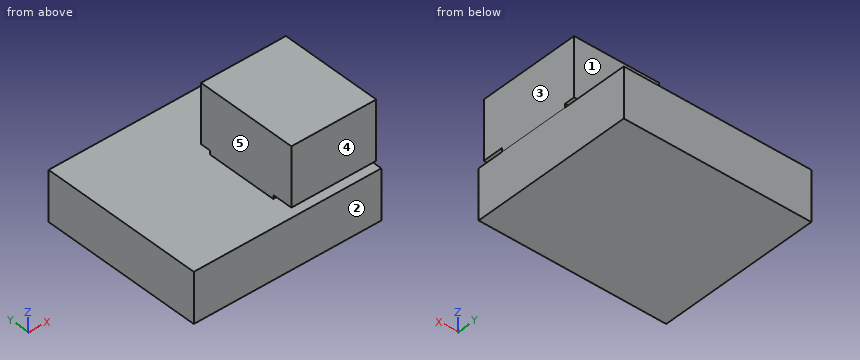
```python
from build123d import *

# Parameters (mm, degrees)
F0_W     = 95.4314470291
F0_H     = 83.3230912685
F1_DEPTH = 25.4
F2_W     = 36.3040966913
F2_H     = 16.6404070333
F3_DEPTH = 43.18


with BuildPart() as f1:
    # F0 (on Top) → F1 (new body)
    with BuildSketch(Plane.XY):
        with Locations((-4.4675134122, -1.5228800476)):
            Rectangle(F0_W, F0_H)
    extrude(amount=F1_DEPTH)

    # F2 (on Right) → F3 (join)
    with BuildSketch(Plane.YZ):
        Polygon((-40.3462946415, 57.2510994971), (-40.3462946415, 27.3906495422), (-29.9596916884, 27.3906495422), (6.3444050029, 27.3906495422), (11.5222530439, 27.3906495422), (11.5222530439, 57.2510994971), align=None)
        with Locations((-11.8076433428, 19.0704460256)):
            Rectangle(F2_W, F2_H)
    extrude(amount=F3_DEPTH)


solid = f1.part
```
Check sheet for the modelled part. Datum: model origin and axes. Units: mm. Face numbers are marked on the shaded views. A direction names the side the tool comes from. Round coordinates to 2 decimals unless told otherwise and drop trailing zeros. Order: outer loops, then holes, each group sorted by start corner. A loop starts at its lowest first (then second) coordinate and runs counter-clockwise, first axis right, second up. Notation, with made-up numbers: M -38.5,-27.5 L 11.5,-27.5 A29 ccw 11.5,1.5 Z; hole C -4.75,27.5 d5. An arc over 180 degrees is marked long. Answer in a Markdown table with one row per item.
(1) Set-up check for the marked faces 1 and 2: record each of +Z, -Z, +X, -X, +Y, -Y from which the full face is reachable in a straight line by a thin tool's end or side.
Findings:
| item | result |
|---|---|
| face 1 | +Z, +X, -X, +Y |
| face 2 | +Z, -Z, +X, -X, -Y |
(2) Section check D-D on z = 46. Record the boundary of the cut face in (x, y), plus the area to 3 significant figures.
Findings:
| item | result |
|---|---|
| outline | M 0,-40.35 L 43.18,-40.35 L 43.18,11.52 L 0,11.52 Z |
| area | 2,240 mm^2 |
(3) Gauge pin test, flat ends, axial feed: pin 1 (16 mm diameter, centred on y = -24.5, z = 43.5, fed in from +X); pin 2 (1 mm diameter, centred on x = 29, z = 26.5, fed in from -Y); pin 3 (16 mm diameter, centred on y = -9.5, z = 43.5, fed in from -X). Record the tip position at first contact, or that the pin passes through.
Findings:
| item | result |
|---|---|
| pin 1 | stops at x = 43.18 |
| pin 2 | stops at y = -29.96 |
| pin 3 | stops at x = 0 |
(4) Draft check along X on the marked faces 3, 4 and 5. Enter one of: +X half, -X half, draft (parallel to the pull), parting line (faces both ways), or undercut.
Findings:
| item | result |
|---|---|
| face 3 | +X half |
| face 4 | draft |
| face 5 | -X half |
(5) Material ranges on line 1 along Z through (x, y) = (18.5, -33.5); line 2 along Z through (x, y) = (-8, -7); line 3 along X through (y, z) = (4, 39.5), recorded low to high. Write a range as from..to.
Findings:
| item | result |
|---|---|
| line 1 | z = 0..25.4, 27.39..57.25 |
| line 2 | z = 0..25.4 |
| line 3 | x = 0..43.18 |
(6) Section check B-B on x = 11. Record the boundary of the cut face in (y, z).
Findings:
| item | result |
|---|---|
| outline | M -43.18,0 L 40.14,0 L 40.14,25.4 L 6.34,25.4 L 6.34,27.39 L 11.52,27.39 L 11.52,57.25 L -40.35,57.25 L -40.35,27.39 L -29.96,27.39 L -29.96,25.4 L -43.18,25.4 Z |
(7) Section check C-C on y = -7. Record the boundary of the cut face in (x, z).
Findings:
| item | result |
|---|---|
| outline | M -52.18,0 L 43.25,0 L 43.25,25.4 L 43.18,25.4 L 43.18,57.25 L 0,57.25 L 0,25.4 L -52.18,25.4 Z |
(8) Section check A-A on y = 9. Record the boundary of the cut face in (x, z).
Findings:
| item | result |
|---|---|
| outline | M -52.18,0 L 43.25,0 L 43.25,25.4 L -52.18,25.4 Z; M 0,27.39 L 43.18,27.39 L 43.18,57.25 L 0,57.25 Z |
